Could you check a few things on this model? Use its own coordinates, in mm. A direction names the side the tool comes from. Give positions to 0.01 mm unless a question says otherwise; leave off trailing zeros. Order: outer loops, then holes, each group sorted by start corner. A loop starts at its lowest first (then second) coordinate and runs counter-clockwise, first axis right, second up.
Autodesk Inventor part; units mm, degrees
ref_plane "YZ Plane" through (0, 0, 0) normal (1, 0, 0) x (0, 1, 0)
ref_plane "XZ Plane" through (0, 0, 0) normal (0, 1, 0) x (-1, 0, 0)
ref_plane "XY Plane" through (0, 0, 0) normal (0, 0, 1) x (1, 0, 0)
ref_plane "Work Plane1" through (-4.987218, -5.774768, 0) normal (0, 0, 1) x (0.9999987, 0.0016281, 0)
sketch "Sketch1" plane through (-4.987218, -5.774768, 0) normal (0, 0, 1) x (0.9999987, 0.0016281, 0)
  circle A0 centre (0.000199, -0.002158) radius 38.1
  circle A1 centre (0.000199, -0.002158) radius 37.8
  circle A2 centre (-0.048773, -0.058769) radius 6.775396
  circle A3 centre (6.079487, 22.963606) radius 1.4
  circle A4 centre (-16.87798, -16.104757) radius 1.4
  circle A5 centre (22.663033, 7.130604) radius 1.4
  point P0 (4.996614, 5.76664)
  dimension "d0" = 0.3
sketch "Sketch1 outline for Extrusion1" plane through (-4.987218, -5.774768, 0) normal (0, 0, 1) x (0.9999987, 0.0016281, 0)
  circle A0 centre (0.000199, -0.002158) radius 37.8
  circle A1 centre (-16.87798, -16.104757) radius 1.4
  circle A2 centre (-0.048773, -0.058769) radius 6.775396
  circle A3 centre (22.663033, 7.130604) radius 1.4
  circle A4 centre (6.079487, 22.963606) radius 1.4
extrude "Extrusion1" add sketch "Sketch1 outline for Extrusion1" along normal blind 5
sketch "Sketch4" plane through (-4.987218, -5.774768, 5) normal (0, 0, 1) x (0.9999987, 0.0016281, 0)
  circle A0 centre (19.372358, 5.196915) radius 1.4
  circle A1 centre (-9.548696, -11.058773) radius 1.352011
  circle A2 centre (-9.548696, -11.058773) radius 3.95399
  point P0 (4.996614, 5.76664)
extrude "Extrusion4" cut sketch "Sketch4" against normal blind 25.4 contours A1 | A2
shell "Shell1" thickness 2.54 removed faces 1 at (15.854163, -10.364044, 0)
properties part number "Anglerfish_3inch_tube_adapterplate_focus"
Item 1: For pin 1 (1.5 mm diameter, centred on y = 10, z = 2, fed in from -X); pin 2 (1.5 mm diameter, centred on x = -18, z = 1.5, fed in from +Y); pin 3 (11 mm diameter, centred on x = -5.04, y = -5.83, fed in from +Z), each with a flat end and sliding along its axis, tell me the tip position at first contact or that it passes through.
Findings:
pin 1: stops at x = -39.67
pin 2: stops at y = 29.98
pin 3: passes through
Item 2: For faces 1 (the flat face through (19.4, 1.5, 0)), 2 (the cylindrical face through (21.424, 0.215, 1.213)), which set-ups out of +Z, -Z, +X, -X, +Y, -Y let a thin tool reach every point of the face, with its end or its side?
Findings:
face 1: -Z, +X, -X, +Y, -Y
face 2: -Z
Item 3: We'd pull the mould along X, two halves only. Please class faces 3 (the cylindrical face through (0.76, 1.46, 1.21)), 4 (the cylindrical face through (-10.45, -21.91, 1.25)), 5 (the cylindrical face through (-32.806, -31.369, 2.465)), 6 (the flat face through (20, -31, 0)): +X half, -X half, draft (parallel to the pull), parting line (faces both ways), or undercut.
Findings:
face 3: undercut
face 4: undercut
face 5: parting line
face 6: draft
Item 4: Please list where these lines run through material, in increasing order: line 1 along Y through (x, z) = (-23, 1.4); line 2 along Y through (x, z) = (-10.5, 1.4); line 3 along X through (y, z) = (14.5, 0.35).
Findings:
line 1: y = -39.01 to -36.09, -25.67 to -22.69, -21.12 to -18.14, 24.53 to 27.46
line 2: y = -43.17 to -40.6, -21.95 to -9.84, -1.83 to 1.71, 29.05 to 31.62
line 3: x = -36.89 to -33.83, -1.82 to 3.93, 23.86 to 26.91
Item 5: Imagine slicing it at A-A on x = -1.5. List the corners of the cut face in (y, z) for me, then the cut area to 3 significant figures.
Findings:
outline: (-43.42, 0) - (-40.86, 0) - (-40.86, 2.46) - (-14.45, 2.46) - (-14.45, 0) - (-11.61, 0) - (-11.61, 5) - (-43.42, 5) - close; (-0.05, 0) - (2.78, 0) - (2.78, 2.46) - (14.2, 2.46) - (14.2, 0) - (20.2, 0) - (20.2, 2.46) - (29.31, 2.46) - (29.31, 0) - (31.86, 0) - (31.86, 5) - (-0.05, 5) - close
area: 203 mm2
Item 6: Imagine slicing it at D-D on x = -34.5. List the corners of the cut face in (y, z) for me.
Findings:
outline: (-29.4, 0) - (-25.07, 0) - (-25.07, 2.46) - (13.52, 2.46) - (13.52, 0) - (17.84, 0) - (17.84, 5) - (-29.4, 5) - close
Item 7: Imagine slicing it at C-C on x = 28. List the corners of the cut face in (y, z) for me, then the cut area to 3 significant figures.
Findings:
outline: (-24.23, 0) - (-18.23, 0) - (-18.23, 2.46) - (6.68, 2.46) - (6.68, 0) - (12.68, 0) - (12.68, 5) - (-24.23, 5) - close
area: 123 mm2
